Read the model definition and answer for the solid it produces. Units are mm, in the model's axes. Face numbers are marked on the shaded views. A direction names the side the tool comes from. Give positions to 0.01 mm unless a question says otherwise; leave off trailing zeros. Order: outer loops, then holes, each group sorted by start corner. A loop starts at its lowest first (then second) coordinate and runs counter-clockwise, first axis right, second up. Notation, with made-up numbers: (42.25, 46.25) - (47.25, 46.25) arc R20 ccw to (47.25, 62.25) - close; hole circle Ø8 at (13, 10.5). An arc over 180 degrees is marked (long way). Use a Markdown table: item, result. Add a question column.
1. Flat-ended cylindrical pins translate along their axes: P1, Ø1.5, axis at y = 13, z = 1.5, coming from the -X side; P2, Ø1, axis at x = 0.5, z = 2, coming from the +Y side; P3, Ø1, axis at x = -1.5, y = 17, coming from the -Z side. Find the tip coordinate at first contact, or state that the pin passes through.
2. A cutting plane is placed at C-C on y = 23. Determine the outline of the cut face in (x, z), and give its area (3 significant figures).
3. A cutting plane is placed at A-A on z = 0. Determine the outline of the cut face in (x, y), and give its area (3 significant figures).
4. A cutting plane is placed at B-B on x = 0. Determine the outline of the cut face in (y, z).
5. A cutting plane is placed at D-D on y = 4. Determine the outline of the cut face in (x, z).
6. Which of the six approach directions +Z, -Z, +X, -X, +Y, -Y give full straight-line access (tool end or side, diameter ignored) to the marked faces 1 and 2?
7. Consider L1, parallel to Y at x = -2.25, z = 1; L2, parallel to Z at x = 2.5, y = 10.75; L3, parallel to Z at x = -1.25, y = 12.25. Determine where each line is inside the solid, lowest interval first.
```python
from build123d import *

# Parameters (mm, degrees)
SKETCH1_R           = 3.5
BOSS_EXTRUDE1_DEPTH = 20
FILLET1_R           = 0.3
SKETCH2_R           = 1
BOSS_EXTRUDE2_DEPTH = 0.3
SKETCH3_R           = 0.5
BOSS_EXTRUDE3_DEPTH = 5
FILLET2_R           = 0.1


with BuildPart() as part:
    # Sketch1 → Boss-Extrude1 (new body)
    with BuildSketch(Plane(origin=(0, 0, 0), x_dir=(1, 0, 0), z_dir=(0, 1, 0))):
        Circle(SKETCH1_R)
    extrude(amount=BOSS_EXTRUDE1_DEPTH)

    # Fillet1
    fillet1_edges = [part.edges().sort_by_distance(p)[0] for p in [
        (-3.5, 20, 0),
    ]]
    fillet(fillet1_edges, radius=FILLET1_R)

    # Sketch2 → Boss-Extrude2 (add)
    with BuildSketch(Plane(origin=(0, 20, 0), x_dir=(1, 0, 0), z_dir=(0, 1, 0))):
        Circle(SKETCH2_R)
    extrude(amount=BOSS_EXTRUDE2_DEPTH)

    # Sketch3 → Boss-Extrude3 (add)
    with BuildSketch(Plane(origin=(0, 20.3, 0), x_dir=(1, 0, 0), z_dir=(0, 1, 0))):
        Circle(SKETCH3_R)
    extrude(amount=BOSS_EXTRUDE3_DEPTH)

    # Fillet2
    fillet2_edges = [part.edges().sort_by_distance(p)[0] for p in [
        (-0.5, 25.3, 0),
    ]]
    fillet(fillet2_edges, radius=FILLET2_R)


solid = part.part
```
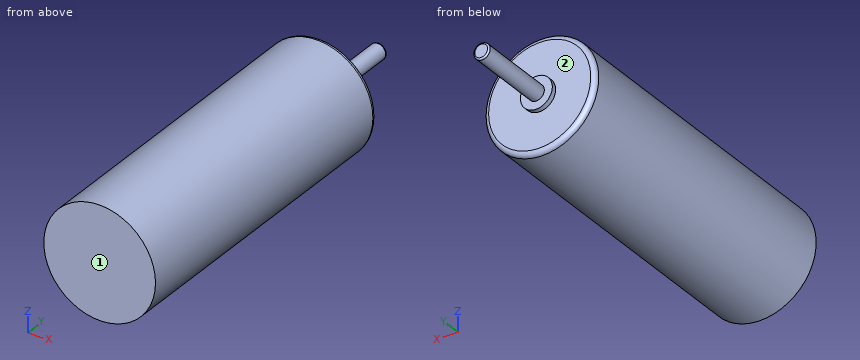
Output values:
| question | item | result |
|---|---|---|
| 1 | P1 | x = -3.42 |
| 1 | P2 | y = 20 |
| 1 | P3 | z = -3.35 |
| 2 | outline | circle Ø1 at (0, 0) |
| 2 | area | 0.785 mm² |
| 3 | outline | (-3.5, 0) - (3.5, 0) - (3.5, 19.7) arc R0.3 ccw to (3.2, 20) - (1, 20) - (1, 20.3) - (0.5, 20.3) - (0.5, 25.2) arc R0.1 ccw to (0.4, 25.3) - (-0.4, 25.3) arc R0.1 ccw to (-0.5, 25.2) - (-0.5, 20.3) - (-1, 20.3) - (-1, 20) - (-3.2, 20) arc R0.3 ccw to (-3.5, 19.7) - close |
| 3 | area | 146 mm² |
| 4 | outline | (0, -3.5) - (19.7, -3.5) arc R0.3 ccw to (20, -3.2) - (20, -1) - (20.3, -1) - (20.3, -0.5) - (25.2, -0.5) arc R0.1 ccw to (25.3, -0.4) - (25.3, 0.4) arc R0.1 ccw to (25.2, 0.5) - (20.3, 0.5) - (20.3, 1) - (20, 1) - (20, 3.2) arc R0.3 ccw to (19.7, 3.5) - (0, 3.5) - close |
| 5 | outline | circle Ø7 at (0, 0) |
| 6 | face 1 | +Z, -Z, +X, -X, -Y |
| 6 | face 2 | +Y |
| 7 | L1 | 0 to 20 |
| 7 | L2 | -2.45 to 2.45 |
| 7 | L3 | -3.27 to 3.27 |
